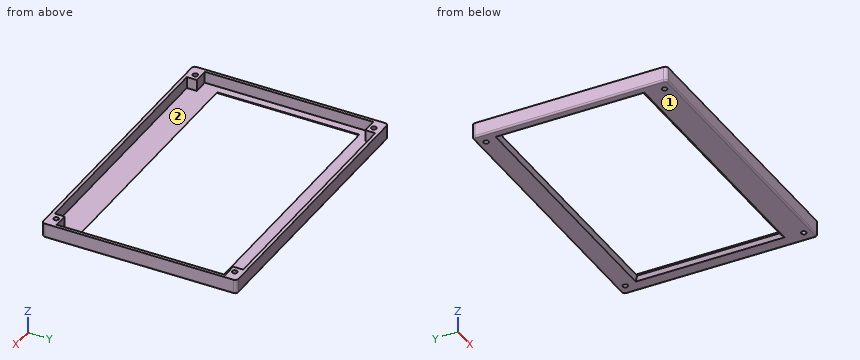
from build123d import *

# Parameters (mm, degrees)
F0_W          = 171
F0_H          = 118
F0_W_2        = 154
F0_H_2        = 86
F1_DEPTH      = 2
F2_SIZE       = 1.99999
F3_R          = 1
F4_W          = 171
F4_H          = 118
F4_W_2        = 167
F4_H_2        = 114
F5_DEPTH      = 7
F6_W          = 9
F6_H          = 6
F7_DEPTH      = 7
F8_R          = 1.525
F9_DEPTH      = 9.001
F10_T1_DEPTH  = 14
F10_T4_ANGLE  = 90
F10_T6_ANGLE  = 90
F10_T8_ANGLE  = 90
F10_T10_ANGLE = 90


# Not quite as in the source:
# - a fillet or chamfer that OpenCascade refuses, or shapes differently, is made with other operations: its cross-section is extruded or revolved along the edge and cut away or added
# - a fillet or chamfer is up to 0.001 mm smaller than in the source, because OpenCascade refuses the exact size


with BuildPart() as f1:
    # F0 (on Top) → F1 (new body)
    with BuildSketch(Plane.XY):
        with Locations((0.75, -1.11)):
            Rectangle(F0_W, F0_H)
        with Locations((-0.75, 1.11)):
            Rectangle(F0_W_2, F0_H_2, mode=Mode.SUBTRACT)
    extrude(amount=-F1_DEPTH)

    # F2 (size 2 in the source; OpenCascade refuses exactly that, so slightly less here)
    f2_edges = [f1.edges().sort_by_distance(p)[0] for p in [
        (76.25, 1.11, -2),
        (-0.75, -41.89, -2),
        (-0.75, 44.11, -2),
        (-77.75, 1.11, -2),
    ]]
    chamfer(f2_edges, length=F2_SIZE)

    # F3
    f3_edges = [f1.edges().sort_by_distance(p)[0] for p in [
        (-84.75, -1.11, -2),
        (0.75, -60.11, -2),
        (86.25, -1.11, -2),
        (0.75, 57.89, -2),
    ]]
    fillet(f3_edges, radius=F3_R)

    # F4 (on face) → F5 (join)
    with BuildSketch(Plane.XY):
        with Locations((0.75, -1.11)):
            Rectangle(F4_W, F4_H)
        with Locations((0.75, -1.11)):
            Rectangle(F4_W_2, F4_H_2, mode=Mode.SUBTRACT)
    extrude(amount=F5_DEPTH)

    # F6 (on face) → F7 (join)
    with BuildSketch(Plane.XY):
        with Locations((-78.25, 52.89)):
            Rectangle(F6_W, F6_H)
        with Locations((79.75, 52.89)):
            Rectangle(F6_W, F6_H)
        with Locations((79.75, -55.11)):
            Rectangle(F6_W, F6_H)
        with Locations((-78.25, -55.11)):
            Rectangle(F6_W, F6_H)
    extrude(amount=F7_DEPTH)

    # F8 (on face) → F9 (cut, through all)
    with BuildSketch(Plane(origin=(0, 0, -2), x_dir=(1, 0, 0), z_dir=(0, 0, -1))):
        with Locations((-77.75, 55.11)):
            Circle(F8_R)
        with Locations((79.25, 55.11)):
            Circle(F8_R)
        with Locations((-77.75, -52.89)):
            Circle(F8_R)
        with Locations((79.25, -52.89)):
            Circle(F8_R)
    extrude(amount=-F9_DEPTH, mode=Mode.SUBTRACT)

    # F10: fillet of radius 2 on 4 edges, made by hand

    # F10_s2 → F10_t1 (cut)
    with BuildSketch(Plane.XY.offset(-2)):
        with BuildLine():
            ThreePointArc((-84.75, 55.89), (-84.1642135624, 57.3042135624), (-82.75, 57.89))
            Line((-82.75, 57.89), (-84.75, 57.89))
            Line((-84.75, 57.89), (-84.75, 55.89))
        make_face()
        with BuildLine():
            ThreePointArc((84.25, 57.89), (85.6642135624, 57.3042135624), (86.25, 55.89))
            Line((86.25, 55.89), (86.25, 57.89))
            Line((86.25, 57.89), (84.25, 57.89))
        make_face()
        with BuildLine():
            ThreePointArc((84.25, -60.11), (85.6642135624, -59.5242135624), (86.25, -58.11))
            Line((86.25, -58.11), (86.25, -60.11))
            Line((86.25, -60.11), (84.25, -60.11))
        make_face()
        with BuildLine():
            ThreePointArc((-84.75, -58.11), (-84.1642135624, -59.5242135624), (-82.75, -60.11))
            Line((-82.75, -60.11), (-84.75, -60.11))
            Line((-84.75, -60.11), (-84.75, -58.11))
        make_face()
    extrude(amount=F10_T1_DEPTH, mode=Mode.SUBTRACT)

    # F10_s3 → F10_t4 (revolve, cut)
    with BuildSketch(Plane.YZ.offset(-82.75)):
        with BuildLine():
            ThreePointArc((-59.11, -2), (-59.8171067812, -1.7071067812), (-60.11, -1))
            Line((-60.11, -1), (-60.11, -2))
            Line((-60.11, -2), (-59.11, -2))
        make_face()
    revolve(axis=Axis((-82.75, -58.11, -2), (0, 0, -1)), revolution_arc=F10_T4_ANGLE, mode=Mode.SUBTRACT)

    # F10_s5 → F10_t6 (revolve, cut)
    with BuildSketch(Plane.XZ.offset(58.11)):
        with BuildLine():
            ThreePointArc((85.25, -2), (85.9571067812, -1.7071067812), (86.25, -1))
            Line((86.25, -1), (86.25, -2))
            Line((86.25, -2), (85.25, -2))
        make_face()
    revolve(axis=Axis((84.25, -58.11, -2), (0, 0, -1)), revolution_arc=F10_T6_ANGLE, mode=Mode.SUBTRACT)

    # F10_s7 → F10_t8 (revolve, cut)
    with BuildSketch(Plane.YZ.offset(84.25)):
        with BuildLine():
            ThreePointArc((56.89, -2), (57.5971067812, -1.7071067812), (57.89, -1))
            Line((57.89, -1), (57.89, -2))
            Line((57.89, -2), (56.89, -2))
        make_face()
    revolve(axis=Axis((84.25, 55.89, -2), (0, 0, -1)), revolution_arc=F10_T8_ANGLE, mode=Mode.SUBTRACT)

    # F10_s9 → F10_t10 (revolve, cut)
    with BuildSketch(Plane.XZ.offset(-55.89)):
        with BuildLine():
            ThreePointArc((-83.75, -2), (-84.4571067812, -1.7071067812), (-84.75, -1))
            Line((-84.75, -1), (-84.75, -2))
            Line((-84.75, -2), (-83.75, -2))
        make_face()
    revolve(axis=Axis((-82.75, 55.89, -2), (0, 0, -1)), revolution_arc=F10_T10_ANGLE, mode=Mode.SUBTRACT)


solid = f1.part
Geometry check sheet. Reference: the model listing, model coordinates, mm. Face numbers are marked on the shaded views. Coordinates: 2 decimals unless noted, no trailing zeros. Loops run counter-clockwise (first coordinate to the right, second up) from the corner with the lowest first, then second, coordinate; pieces in that order, holes last. Notation, with made-up numbers: (68.5, 76.5) - (115.5, 76.5) arc R20 cw to (115.5, 102.5) - close; hole circle Ø1 at (-20, 75.5). An arc over 180 degrees is marked (long way). Use one line per item in the form item = value. Start each with the question number.
Item 1: Mould release check, pull along X, two halves, no side actions. Record for the marked faces 1 and 2: +X half, -X half, draft (parallel to the pull), parting line (faces both ways), or undercut.
Item 2: Thickness scan on probe 1 along Y at (x, z) = (79.25, 1.25) (3 decimals); probe 2 along X at (y, z) = (-55.11, 0.25) (3 decimals); probe 3 along X at (y, z) = (-6.5, 4.5). Record the ranges inside material, lowest first.
Item 3: Section check C-C, the plane z = 1.75. Enter the section's corners in (x, y) (3 decimals), and give its area (3 significant figures).
Computed:
q1.face_1 = draft
q1.face_2 = undercut
q2.probe_1 = -60.11 to -56.635, -53.585 to -52.11, 49.89 to 51.365, 54.415 to 57.89
q2.probe_2 = -84.75 to -79.275, -76.225 to -73.75, 75.25 to 77.725, 80.775 to 86.25
q2.probe_3 = -84.75 to -82.75, 84.25 to 86.25
q3.outline = (-84.75, -58.11) arc R2 ccw to (-82.75, -60.11) - (84.25, -60.11) arc R2 ccw to (86.25, -58.11) - (86.25, 55.89) arc R2 ccw to (84.25, 57.89) - (-82.75, 57.89) arc R2 ccw to (-84.75, 55.89) - close; hole (-82.75, -52.11) - (-73.75, -52.11) - (-73.75, -58.11) - (75.25, -58.11) - (75.25, -52.11) - (84.25, -52.11) - (84.25, 49.89) - (75.25, 49.89) - (75.25, 55.89) - (-73.75, 55.89) - (-73.75, 49.89) - (-82.75, 49.89) - close; hole circle Ø3.05 at (-77.75, -55.11); hole circle Ø3.05 at (-77.75, 52.89); hole circle Ø3.05 at (79.25, -55.11); hole circle Ø3.05 at (79.25, 52.89)
q3.area = 1,320 mm2
